Verification items for the finished model (mm, model axes). Round coordinates to 2 decimals unless told otherwise and drop trailing zeros. Order: outer loops, then holes, each group sorted by start corner. A loop starts at its lowest first (then second) coordinate and runs counter-clockwise, first axis right, second up. Notation, with made-up numbers: M 14.25,23 L 56.25,23 A15 cw 56.25,50 Z; hole C -22.5,5.5 d6. An arc over 180 degrees is marked long. Use one line per item in the form item = value. Start each with the question number.
Item 1: Cross-section at C-C on z = -15. Enter the section's corners in (x, y) (3 decimals), then the cut area to 3 significant figures.
Item 2: Go/stop test with a flat-tipped pin: pin 1 Ø6 at (x, z) = (-84.5, -45.5) entering from -Y. Record where the tip stops, or that it passes through.
Item 3: Cross-section at B-B on x = -71.75. Enter the section's corners in (y, z).
Item 4: Cross-section at A-A on z = -32. Enter the section's corners in (x, y) (3 decimals).
Item 5: Cross-section at D-D on y = 2.9. Count the separate pieces of the cut face and the enclosed holes in it, then the cut area to 3 significant figures.
Item 6: Thickness scan on probe 1 along X at (y, z) = (2.1, -104.2); probe 2 along Z at (x, y) = (-46.75, 1.3); probe 3 along X at (y, z) = (2.8, -18.5) (3 decimals). Record the ranges inside material, lowest first. Write a range as [from, to].
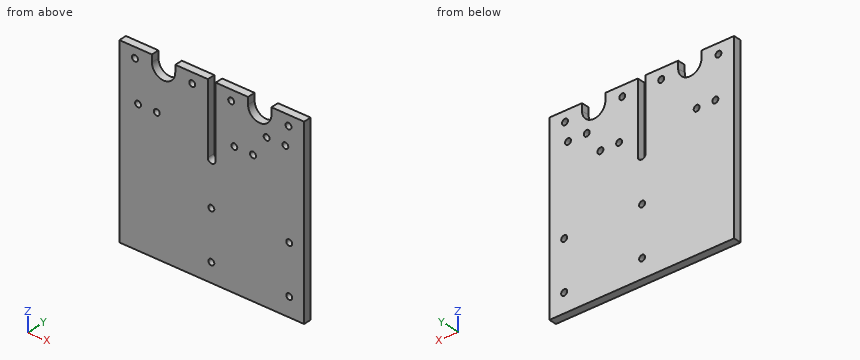
Autodesk Inventor part; units mm, degrees
ref_plane "YZ Plane" through (0, 0, 0) normal (1, 0, 0) x (0, 1, 0)
ref_plane "XZ Plane" through (0, 0, 0) normal (0, 1, 0) x (-1, 0, 0)
ref_plane "XY Plane" through (0, 0, 0) normal (0, 0, 1) x (1, 0, 0)
sketch "Sketch1" plane through (0, 0, 0) normal (0, 1, 0) x (-1, 0, 0)
  line L0 (0, 0) -> (118.5, 0)
  line L1 (118.5, 0) -> (118.5, -116.2)
  line L2 (118.5, -116.2) -> (0, -116.2)
  line L3 (0, -116.2) -> (0, 0)
  dimension "d0" = 118.5
  dimension "d1" = 116.2
extrude "Extrusion1" add sketch "Sketch1" along normal blind 5
sketch "Sketch2" plane through (0, 5, 0) normal (0, 1, 0) x (1, 0, 0)
  line L0 (-59.5, 73.2) -> (-9.5, 73.2)
  line L1 (-9.5, 73.2) -> (-9.5, 104.2)
  line L2 (-9.5, 104.2) -> (-59.5, 104.2)
  line L3 (-59.5, 104.2) -> (-59.5, 73.2)
  line L4 (0, 116.2) -> (-118.5, 116.2)
  line L5 (-118.5, 116.2) -> (-118.5, 0)
  point P0 (0, 0)
  dimension "d4" = 12
  dimension "d5" = 31
  dimension "d6" = 50
  dimension "d7" = 59
hole "Hole1" at (-59.5, 5, -73.2) at (-9.5, 5, -73.2) at (-59.5, 5, -104.2) at (-9.5, 5, -104.2) direction (0, -1, 0) diameter 3.8 end through all
sketch "Sketch3" plane through (0, 5, 0) normal (0, 1, 0) x (1, 0, 0)
  line L0 (-59.25, -19.9196) -> (-59.25, 121.041) construction
  line L1 (-118.5, 0) -> (0, 0)
  line L2 (-61.775, 0) -> (-56.725, 0)
  line L3 (-56.725, 0) -> (-56.725, 45)
  line L4 (-61.775, 45) -> (-61.775, 0)
  arc A0 (-56.725, 45) -> (-61.775, 45) centre (-59.25, 45) ccw
  point P0 (-59.25, 0)
  dimension "d18" = 5.05
  dimension "d19" = 45
extrude "Extrusion2" cut sketch "Sketch3" against normal blind 10
sketch "Sketch4" plane through (0, 5, 0) normal (0, 1, 0) x (1, 0, 0)
  line L0 (-148.0192, 32) -> (31.7399, 32) construction
  line L1 (-56.725, 0) -> (0, 0) construction
  line L2 (-118.5, 116.2) -> (-118.5, 0) construction
  line L3 (-59.25, 61.4977) -> (-59.25, -14.0332) construction
  line L4 (-61.775, 45) -> (-61.775, 0) construction
  arc A0 (-56.725, 45) -> (-61.775, 45) centre (-59.25, 45) ccw construction
  line L5 (-27.032, 18.5) -> (18.1948, 18.5) construction
  line L6 (0, 0) -> (0, 116.2) construction
  point P0 (-106.5, 32)
  point P1 (-94.5, 32)
  point P2 (-44.75, 32)
  point P3 (-32.75, 32)
  point P4 (-59.25, 47.525)
  point P5 (-12, 18.5)
  point P6 (-24, 18.5)
  dimension "d22" = 32
  dimension "d23" = 12
  dimension "d24" = 12
  dimension "d25" = 12
  dimension "d26" = 14.5
  dimension "d27" = 18.5
  dimension "d28" = 12
  dimension "d29" = 12
hole "Hole2" at (-106.5, 5, -32) at (-94.5, 5, -32) at (-44.75, 5, -32) at (-32.75, 5, -32) at (-12, 5, -18.5) at (-24, 5, -18.5) direction (0, -1, 0) diameter 3.8 end through all
sketch "Sketch5" plane through (0, 5, 0) normal (0, 1, 0) x (1, 0, 0)
  line L0 (-134.8767, 6.5) -> (26.057, 6.5) construction
  line L1 (-56.725, 0) -> (0, 0) construction
  line L2 (0, 0) -> (0, 116.2) construction
  line L3 (-118.5, 116.2) -> (-118.5, 0) construction
  line L4 (-59.25, 58.1) -> (-59.25, -13.4303) construction
  arc A0 (-56.725, 45) -> (-61.775, 45) centre (-59.25, 45) ccw construction
  point P0 (-108.5, 6.5)
  point P1 (-71.75, 6.5)
  point P2 (-46.75, 6.5)
  point P3 (-10, 6.5)
  point P4 (-59.25, 47.525)
  dimension "d37" = 6.5
  dimension "d38" = 10
  dimension "d39" = 10
  dimension "d40" = 12.5
  dimension "d41" = 12.5
hole "Hole3" at (-108.5, 5, -6.5) at (-71.75, 5, -6.5) at (-46.75, 5, -6.5) at (-10, 5, -6.5) direction (0, -1, 0) diameter 3.8 end through all
sketch "Sketch6" plane through (0, 5, 0) normal (0, 1, 0) x (1, 0, 0)
  line L0 (-90.1375, 21.1453) -> (-90.1375, -29.1073) construction
  line L1 (-28.4418, 11.0948) -> (-28.4418, -20.2874) construction
  line L2 (-90.1375, -5.5) -> (-90.1375, 4.5) construction
  line L3 (-82.6375, -5.5) -> (-82.6375, 4.5)
  line L4 (-97.6375, 4.5) -> (-97.6375, -5.5)
  arc A0 (-97.6375, -5.5) -> (-82.6375, -5.5) centre (-90.1375, -5.5) ccw
  arc A1 (-82.6375, 4.5) -> (-97.6375, 4.5) centre (-90.1375, 4.5) ccw
  line L5 (-28.4418, -5.5) -> (-28.4418, 4.5) construction
  line L6 (-20.9418, -5.5) -> (-20.9418, 4.5)
  line L7 (-35.9418, 4.5) -> (-35.9418, -5.5)
  arc A2 (-35.9418, -5.5) -> (-20.9418, -5.5) centre (-28.4418, -5.5) ccw
  arc A3 (-20.9418, 4.5) -> (-35.9418, 4.5) centre (-28.4418, 4.5) ccw
  line L8 (-56.725, 0) -> (0, 0)
  line L9 (-118.5, 0) -> (-61.775, 0)
  line L10 (-118.5, 0) -> (-61.775, 0)
  line L11 (-97.6375, 0) -> (-82.6375, 0)
  line L12 (-35.9418, 0) -> (-20.9418, 0)
  point P0 (-90.1375, -0.5)
  point P1 (-28.4418, -0.5)
  point P2 (-97.6375, 0)
  point P3 (-82.6375, 0)
  dimension "d49" = 15
  dimension "d50" = 15
  dimension "d51" = 4.5
  dimension "d52" = 4.5
  dimension "d53" = 10
  dimension "d54" = 10
extrude "Extrusion3" cut sketch "Sketch6" against normal through all contours L9 L4 A1 L3 | L8 L7 A3 L6
properties part number "Battery Base Plate"
Output values:
q1.outline = M -118.5,0 L -61.775,0 L -61.775,5 L -118.5,5 Z; M -56.725,0 L 0,0 L 0,5 L -56.725,5 Z
q1.area = 567 mm2
q2.pin_1 = 0
q3.outline = M 0,-116.2 L 5,-116.2 L 5,-8.4 L 0,-8.4 Z; M 0,-4.6 L 5,-4.6 L 5,0 L 0,0 Z
q4.outline = M -118.5,0 L -108.4,0 L -108.4,5 L -118.5,5 Z; M -104.6,0 L -96.4,0 L -96.4,5 L -104.6,5 Z; M -92.6,0 L -61.775,0 L -61.775,5 L -92.6,5 Z; M -56.725,0 L -46.65,0 L -46.65,5 L -56.725,5 Z; M -42.85,0 L -34.65,0 L -34.65,5 L -42.85,5 Z; M -30.85,0 L 0,0 L 0,5 L -30.85,5 Z
q5.separate_pieces = 1
q5.enclosed_holes = 14
q5.area = 13,100 mm2
q6.probe_1 = [-118.5, -61.4], [-57.6, -11.4], [-7.6, 0]
q6.probe_2 = [-116.2, -8.4], [-4.6, 0]
q6.probe_3 = [-118.5, -61.775], [-56.725, -25.9], [-22.1, -13.9], [-10.1, 0]
